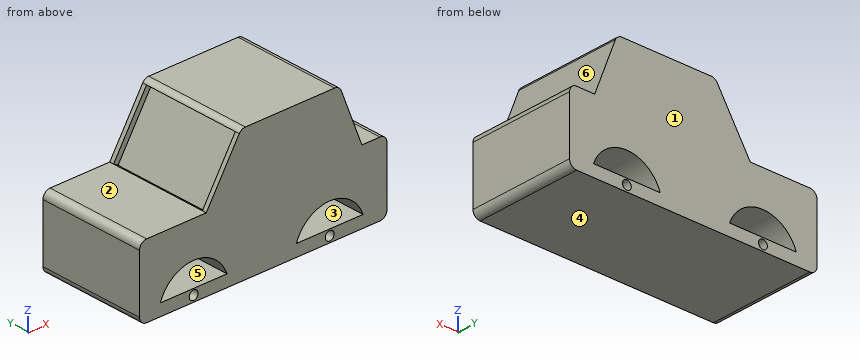
from build123d import *

# Parameters (mm, degrees)
F0_W      = 177.8
F0_H      = 76.2
F1_DEPTH  = 101.6
F3_DEPTH  = 203.2
F4_R      = 5.08
F5_W      = 70.067029912
F5_H      = 45.8034253509
F6_DEPTH  = 3.81
F8_DEPTH  = 203.2
F10_DEPTH = 76.2
F11_R     = 3.175
F12_DEPTH = 76.2


with BuildPart() as f1:
    # F0 (on Top) → F1 (new body)
    with BuildSketch(Plane.XY):
        with Locations((88.9, -38.1)):
            Rectangle(F0_W, F0_H)
    extrude(amount=F1_DEPTH)

    # F2 (on face) → F3 (cut)
    with BuildSketch(Plane.XZ.offset(76.2)):
        Polygon((0, 101.6), (0, 50.8), (47.9459241033, 50.8), (73.1289312243, 92.4461781979), (143.6413377523, 92.4461781979), (159.7584486008, 50.8), (177.8, 50.8), (177.8, 101.6), align=None)
    extrude(amount=-F3_DEPTH, mode=Mode.SUBTRACT)

    # F4
    f4_edges = [f1.edges().sort_by_distance(p)[0] for p in [
        (0, -38.1, 50.8),
        (73.128931, -38.1, 92.446178),
        (143.641338, -38.1, 92.446178),
        (177.8, -38.1, 50.8),
        (177.8, -38.1, 0),
        (0, -38.1, 0),
    ]]
    fillet(f4_edges, radius=F4_R)

    # F5 (on face) → F6 (cut)
    with BuildSketch(Plane(origin=(12.6150217606, 0, -7.6281713371), x_dir=(0, -1, 0), z_dir=(-0.8557174536, 0, 0.5174433684))):
        with Locations((38.0591393914, 91.1814597909)):
            Rectangle(F5_W, F5_H)
    extrude(amount=-F6_DEPTH, mode=Mode.SUBTRACT)

    # F7 (on face) → F8 (cut)
    with BuildSketch(Plane.XZ.offset(76.2)):
        with BuildLine():
            ThreePointArc((162.0320997477, 0), (136.6320997477, 25.4), (111.2320997477, 0))
            Line((111.2320997477, 0), (162.0320997477, 0))
        make_face()
        with BuildLine():
            Line((13.4567559421, 0), (64.2567559421, 0))
            ThreePointArc((64.2567559421, 0), (38.8567559421, 25.4), (13.4567559421, 0))
        make_face()
    extrude(amount=-F8_DEPTH, mode=Mode.SUBTRACT)

    # F9 (on face) → F10 (join)
    with BuildSketch(Plane(origin=(0, 0, 0), x_dir=(-1, 0, 0), z_dir=(0, 1, 0))):
        with BuildLine():
            ThreePointArc((-160.5904804881, 8.4354011342), (-161.6691010738, 4.2788508499), (-162.0320997477, 0))
            Line((-162.0320997477, 0), (-111.2320997477, 0))
            ThreePointArc((-111.2320997477, 0), (-111.5950984215, 4.2788508499), (-112.6737190072, 8.4354011342))
            Line((-112.6737190072, 8.4354011342), (-160.5904804881, 8.4354011342))
        make_face()
        with BuildLine():
            ThreePointArc((-62.8151366826, 8.4354011342), (-63.8937572682, 4.2788508499), (-64.2567559421, 0))
            Line((-64.2567559421, 0), (-13.4567559421, 0))
            ThreePointArc((-13.4567559421, 0), (-13.819754616, 4.2788508499), (-14.8983752016, 8.4354011342))
            Line((-14.8983752016, 8.4354011342), (-62.8151366826, 8.4354011342))
        make_face()
    extrude(amount=-F10_DEPTH)

    # F11 (on face) → F12 (cut)
    with BuildSketch(Plane.XZ.offset(76.2)):
        with Locations((38.8567559421, 4.3010804802)):
            Circle(F11_R)
        with Locations((136.6320997477, 4.3010804802)):
            Circle(F11_R)
    extrude(amount=-F12_DEPTH, mode=Mode.SUBTRACT)


solid = f1.part
Can you work these out from the model? Positions are in its coordinate system, mm. Face numbers are marked on the shaded views. A direction names the side the tool comes from. Give positions to 0.01 mm unless a question says otherwise; leave off trailing zeros. Order: outer loops, then holes, each group sorted by start corner. A loop starts at its lowest first (then second) coordinate and runs counter-clockwise, first axis right, second up. Notation, with made-up numbers: M 29,55 L 64,55 A31 ccw 64,88 Z; hole C -16,61 d4. An arc over 180 degrees is marked long. Use one line per item in the form item = value. Start each with the question number.
Item 1: If I drill on line 1 along X through (y, z) = (-33, 17.5); line 2 along X through (y, z) = (-51, 22); line 3 along Z through (x, y) = (127, -42), over which ranges is the centre line in solid material (lowest first)?
Item 2: We'd pull the mould along Z, two halves only. Please class the marked faces 4, 5 and 6: +Z half, -Z half, draft (parallel to the pull), parting line (faces both ways), or undercut.
Item 3: If we section it at A-A (x = 151): Write out the boundary of the cut face in (y, z), then the cut area to 3 significant figures.
Item 4: If we section it at D-D (z = 55.5): Write out the boundary of the cut face in (x, y).
Item 5: Will these pins go through, and if not, where does the flat tip stop? pin 1 Ø6.5 at (x, y) = (169, -44.5) entering from +Z; pin 2 Ø1 at (y, z) = (-58, 53) entering from -X; pin 3 Ø10 at (y, z) = (-68, 58.5) entering from +X.
Item 6: If we section it at C-C (y = -19.5): Write out the boundary of the cut face in (x, z) (3 decimals), then the cut area to 3 significant figures.
Item 7: If we section it at B-B (z = 19): Write out the boundary of the cut face in (x, y), then the cut area to 3 significant figures.
Item 8: For the marked faces 1, 2 and 3, which set-ups out of +Z, -Z, +X, -X, +Y, -Y let a thin tool reach every point of the face, with its end or its side?
Outcome:
q1.line_1 = 0 to 20.45, 57.27 to 118.22, 155.04 to 177.8
q1.line_2 = 0 to 26.16, 51.55 to 123.94, 149.33 to 177.8
q1.line_3 = 0 to 8.44, 23.5 to 92.45
q2.face_4 = -Z half
q2.face_5 = undercut
q2.face_6 = +Z half
q3.outline = M -76.2,0 L 0,0 L 0,8.44 L -76.2,8.44 Z; M -76.2,20.95 L 0,20.95 L 0,73.43 L -76.2,73.43 Z
q3.area = 4,640 mm2
q4.outline = M 50.79,-76.2 L 157.94,-76.2 L 157.94,0 L 50.79,0 L 50.79,-3.03 L 55.24,-3.03 L 55.24,-73.09 L 50.79,-73.09 Z
q5.pin_1 = 50.8
q5.pin_2 = 53.43
q5.pin_3 = 158.71
q6.outline = M 0,5.08 A5.08 ccw 5.08,0 L 172.72,0 A5.08 ccw 177.8,5.08 L 177.8,45.72 A5.08 ccw 172.72,50.8 L 159.758,50.8 L 144.898,89.2 A5.08 ccw 140.16,92.446 L 75.994,92.446 A5.08 ccw 71.647,89.995 L 74.907,88.023 L 51.206,48.829 L 47.946,50.8 L 5.08,50.8 A5.08 ccw 0,45.72 Z; hole M 14.898,8.435 L 62.815,8.435 A25.4 ccw Z; hole C 38.857,4.301 d6.35; hole M 112.674,8.435 L 160.59,8.435 A25.4 ccw Z; hole C 136.632,4.301 d6.35
q6.area = 11,400 mm2
q7.outline = M 0,-76.2 L 22,-76.2 L 22,0 L 0,0 Z; M 55.71,-76.2 L 119.78,-76.2 L 119.78,0 L 55.71,0 Z; M 153.49,-76.2 L 177.8,-76.2 L 177.8,0 L 153.49,0 Z
q7.area = 8,410 mm2
q8.face_1 = +Z, -Z, +X, -X, +Y
q8.face_2 = +Z, -X, +Y, -Y
q8.face_3 = +Y, -Y
